Build history of the part. All positions in model axes, mm. A direction names the side the tool comes from. Give positions to 0.01 mm unless a question says otherwise; leave off trailing zeros. Order: outer loops, then holes, each group sorted by start corner. A loop starts at its lowest first (then second) coordinate and runs counter-clockwise, first axis right, second up. Notation, with made-up numbers: (-31.75, -15.75) -> (23.25, -15.75) arc R36 ccw to (23.25, 20.25) -> close; hole circle Ø6 at (35.5, 88.25). An arc over 180 degrees is marked (long way). One line per item, written item: value. Start each with the question number.
(1) Saw through at A-A on x = 7. Give the cut face in (y, z).
(2) Saw through at B-B on y = 15. Give the cut face in (x, z).
(3) Two-plate mould, pull along Y, no slides. Class faces 1 (the cylindrical face through (-15, -0.1, 9.5)), 2 (the cylindrical face through (21, -25, 8)), 3 (the cylindrical face through (-8.65, -17.93, 7.04)), 4 (the flat face through (-30, 0, 5)): +Y half, -Y half, draft (parallel to the pull), parting line (faces both ways), or undercut.
(4) Saw through at D-D on z = 6.25. Count the separate pieces of the cut face and the enclosed holes in it, plus the area to 3 significant figures.
(5) Pin check, flat tips, straight feed: pin 1 (3 mm diameter, centred on x = 2, y = 12.5, fed in from -Z); pin 2 (0.9 mm diameter, centred on x = 27.5, z = 8.5, fed in from +Y); pin 3 (2.5 mm diameter, centred on y = 31, z = 9, fed in from -X). Stop position of each tip, or through.
(6) Saw through at C-C on z = 2.75. Give the cut face in (x, y).
(7) Which spindle directions (+Z, -Z, +X, -X, +Y, -Y) get a long thin tool onto all of the face, cutting with end or side? Do faces 5 (the flat face through (-19, -32, 8)), 6 (the flat face through (11, -22.5, 2)), 7 (the flat face through (26, -29, 7)), 8 (the flat face through (-23, 0, 9)). Say none if no direction does.
(8) Probe line 1 (Y direction, x = 24, z = 2.75); line 2 (Y direction, x = -7, z = 3.75); line 3 (Y direction, x = -8, z = 8.05). List the from-to ranges inside material, lowest first.
```python
from build123d import *

# Parameters (mm, degrees)
SKETCH_1_W          = 60
SKETCH_1_H          = 70
EXTRUDE_1_DEPTH     = 10
SKETCH_2_R          = 3
CUT_EXTRUDE_1_DEPTH = 48.16990566
CUT_EXTRUDE_START   = -4
SKETCH_3_R          = 7.5
SKETCH_3_R_2        = 3
CUT_EXTRUDE_2_DEPTH = 4
SKETCH_4_R          = 5
CUT_EXTRUDE_3_DEPTH = 1
EXTRUDE_2_DEPTH     = 12.5
SKETCH_7_R          = 9.5
CUT_EXTRUDE_4_DEPTH = 12.5
CUT_EXTRUDE_5_DEPTH = 56
SKETCH_9_R          = 1.5
CUT_EXTRUDE_6_DEPTH = 48.16990566
CUT_EXTRUDE_START_2 = -3
SKETCH_10_R         = 1.5
CUT_EXTRUDE_7_DEPTH = 3


with BuildPart() as part:
    # 草图1 → 凸台-拉伸1 (new body)
    with BuildSketch(Plane.XY):
        Rectangle(SKETCH_1_W, SKETCH_1_H)
    extrude(amount=EXTRUDE_1_DEPTH)

    # 草图2 → 切除-拉伸1 (cut, through all)
    with BuildSketch(Plane.XY.offset(10)):
        with Locations((-8, 15)):
            Circle(SKETCH_2_R)
        with Locations((7, 15)):
            Circle(SKETCH_2_R)
        with Locations((-8, -15)):
            Circle(SKETCH_2_R)
        with Locations((7, -15)):
            Circle(SKETCH_2_R)
        with Locations((22, 15)):
            Circle(SKETCH_2_R)
        with Locations((22, -15)):
            Circle(SKETCH_2_R)
    extrude(amount=-CUT_EXTRUDE_1_DEPTH, mode=Mode.SUBTRACT)

    # 草图3 → 切除-拉伸2 (cut)
    # profile 1 of 2: a face of its own
    with BuildSketch(Plane(origin=(0, 0, 0), x_dir=(-1, 0, 0), z_dir=(0, 0, -1)).offset(CUT_EXTRUDE_START)):
        with Locations((8, 15)):
            Circle(SKETCH_3_R)
        with Locations(Location((8, 15, 0), (0, 0, 180))):
            Circle(SKETCH_3_R_2, mode=Mode.SUBTRACT)
    # profile 2 of 2: a face of its own
    with BuildSketch(Plane(origin=(0, 0, 0), x_dir=(-1, 0, 0), z_dir=(0, 0, -1)).offset(CUT_EXTRUDE_START)):
        with BuildLine():
            ThreePointArc((8, 7.5), (0.5, 15), (8, 22.5))
            Line((8, 22.5), (-30, 22.5))
            Line((-30, 22.5), (-30, 7.5))
            Line((-30, 7.5), (8, 7.5))
        make_face()
        with Locations(Location((-7, 15, 0), (0, 0, 180))):
            Circle(SKETCH_3_R_2, mode=Mode.SUBTRACT)
    cut_extrude_2 = extrude(amount=CUT_EXTRUDE_2_DEPTH, mode=Mode.SUBTRACT)

    # 镜向1: 切除-拉伸2 across plane
    add(cut_extrude_2.mirror(Plane.ZX), mode=Mode.SUBTRACT)

    # 草图4 → 切除-拉伸3 (cut)
    with BuildSketch(Plane.XY.offset(10)):
        with Locations((-20, 0)):
            Circle(SKETCH_4_R)
        with BuildLine():
            ThreePointArc((-20, -5), (-25, 0), (-20, 5))
            Line((-20, 5), (-30, 5))
            Line((-30, 5), (-30, -5))
            Line((-30, -5), (-20, -5))
        make_face()
    extrude(amount=-CUT_EXTRUDE_3_DEPTH, mode=Mode.SUBTRACT)

    # 草图6 → 凸台-拉伸2 (add)
    with BuildSketch(Plane(origin=(0, 35, 0), x_dir=(1, 0, 0), z_dir=(0, 1, 0))):
        with BuildLine():
            ThreePointArc((30, 0), (20.807611845, 3.807611845), (17, 13))
            ThreePointArc((17, 13), (0, 30), (-17, 13))
            ThreePointArc((-17, 13), (-20.807611845, 3.807611845), (-30, 0))
            Line((-30, 0), (30, 0))
        make_face()
    extrude_2 = extrude(amount=-EXTRUDE_2_DEPTH)

    # 草图7 → 切除-拉伸4 (cut)
    with BuildSketch(Plane(origin=(0, 35, 0), x_dir=(1, 0, 0), z_dir=(0, 1, 0))):
        with Locations(Location((0, 13, 0), (0, 0, 270))):
            Circle(SKETCH_7_R)
    cut_extrude_4 = extrude(amount=-CUT_EXTRUDE_4_DEPTH, mode=Mode.SUBTRACT)

    # 镜向2: 凸台-拉伸2, 切除-拉伸4 across plane
    add(extrude_2.mirror(Plane.ZX))
    add(cut_extrude_4.mirror(Plane.ZX), mode=Mode.SUBTRACT)

    # 草图8 → 切除-拉伸5 (cut, through all)
    with BuildSketch(Plane(origin=(0, 0, 0), x_dir=(-1, 0, 0), z_dir=(0, 0, -1))):
        with BuildLine():
            Line((30, -5), (20, -5))
            ThreePointArc((20, -5), (15, 0), (20, 5))
            Line((20, 5), (30, 5))
            Line((30, 5), (30, 35))
            Line((30, 35), (-30, 35))
            Line((-30, 35), (-30, -35))
            Line((-30, -35), (30, -35))
            Line((30, -35), (30, -5))
        make_face()
    extrude(amount=CUT_EXTRUDE_5_DEPTH, mode=Mode.SUBTRACT)

    # 草图9 → 切除-拉伸6 (cut, through all)
    with BuildSketch(Plane(origin=(0, 0, 0), x_dir=(-1, 0, 0), z_dir=(0, 0, -1))):
        with Locations((-24, -29)):
            Circle(SKETCH_9_R)
        with Locations((24, -29)):
            Circle(SKETCH_9_R)
    cut_extrude_6 = extrude(amount=-CUT_EXTRUDE_6_DEPTH, mode=Mode.SUBTRACT)

    # 草图10 → 切除-拉伸7 (cut)
    # profile 1 of 2: a face of its own
    with BuildSketch(Plane.XY.offset(10).offset(CUT_EXTRUDE_START_2)):
        with BuildLine():
            Line((-24, -24), (-30, -24))
            Line((-30, -24), (-30, -35))
            Line((-30, -35), (-19, -35))
            Line((-19, -35), (-19, -29))
            ThreePointArc((-19, -29), (-20.464466094, -25.464466094), (-24, -24))
        make_face()
        with Locations(Location((-24, -29, 0), (0, 0, 180))):
            Circle(SKETCH_10_R, mode=Mode.SUBTRACT)
    # profile 2 of 2: a face of its own
    with BuildSketch(Plane.XY.offset(10).offset(CUT_EXTRUDE_START_2)):
        with BuildLine():
            Line((19, -29), (19, -35))
            Line((19, -35), (30, -35))
            Line((30, -35), (30, -24))
            Line((30, -24), (24, -24))
            ThreePointArc((24, -24), (20.464466094, -25.464466094), (19, -29))
        make_face()
        with Locations(Location((24, -29, 0), (0, 0, 180))):
            Circle(SKETCH_10_R, mode=Mode.SUBTRACT)
    cut_extrude_7 = extrude(amount=CUT_EXTRUDE_7_DEPTH, mode=Mode.SUBTRACT)

    # 镜向3: 切除-拉伸6, 切除-拉伸7 across plane
    add(cut_extrude_6.mirror(Plane.ZX), mode=Mode.SUBTRACT)
    add(cut_extrude_7.mirror(Plane.ZX), mode=Mode.SUBTRACT)


solid = part.part
```
Results below:
1. outline: (-35, 0) -> (-22.5, 0) -> (-22.5, 4) -> (-18, 4) -> (-18, 10) -> (-35, 10) -> close; (-12, 4) -> (-7.5, 4) -> (-7.5, 0) -> (7.5, 0) -> (7.5, 4) -> (12, 4) -> (12, 10) -> (-12, 10) -> close; (18, 4) -> (22.5, 4) -> (22.5, 0) -> (35, 0) -> (35, 10) -> (18, 10) -> close
2. outline: (-30, 0) -> (-15.5, 0) -> (-15.5, 4) -> (-11, 4) -> (-11, 10) -> (-30, 10) -> close; (-5, 4) -> (4, 4) -> (4, 10) -> (-5, 10) -> close; (10, 4) -> (19, 4) -> (19, 10) -> (10, 10) -> close; (25, 4) -> (30, 4) -> (30, 10) -> (25, 10) -> close
3. face 1: undercut
3. face 2: -Y half
3. face 3: undercut
3. face 4: draft
4. separate pieces: 1
4. enclosed holes: 10
4. area: 4,000 mm²
5. pin 1: stops at z = 4
5. pin 2: stops at y = 24
5. pin 3: stops at x = -19
6. outline: (-30, -35) -> (30, -35) -> (30, -22.5) -> (-8, -22.5) arc R7.5 cw to (-8, -7.5) -> (30, -7.5) -> (30, 7.5) -> (-8, 7.5) arc R7.5 cw to (-8, 22.5) -> (30, 22.5) -> (30, 35) -> (-30, 35) -> close; hole circle Ø3 at (-24, -29); hole circle Ø3 at (-24, 29); hole circle Ø3 at (24, -29); hole circle Ø3 at (24, 29)
7. face 5: +Z, -X, -Y
7. face 6: -Z, +X
7. face 7: +Z, +X, -Y
7. face 8: +Z, -X
8. line 1: y = -35 to -30.5, -27.5 to -22.5, -7.5 to 7.5, 22.5 to 27.5, 30.5 to 35
8. line 2: y = -35 to -22.5, -7.5 to 7.5, 22.5 to 35
8. line 3: y = -35 to -18, -12 to 12, 18 to 35
